Geometry: see drawing. Coordinates: mm, zero at the bounding-box minimum. A direction names the side the tool comes from. Coordinates: 2 decimals unless noted, no trailing zeros. Write each loop counter-clockwise with the first axis right and the second up, starting at its lowest first coordinate (ties: lowest second). Pieces come first, ordered by that corner, then holes. Notation, with made-up numbers: M 66.5,9.25 L 105.5,9.25 A31 ccw 105.5,38.25 Z; hole C 70,87 d10. An arc over 180 degrees is marked long. One line per item, written item: value. Start each with the question number.
Item 1: Cut plane B-B, the plane y = 17. Output: boundary loops of the cut face in (x, z), then the cut area to 3 significant figures.
Item 2: Mould query, pull axis Z, two halves, no side actions, for the marked faces 5, 6 and 7. Classes: released by +Z, released by -Z, zero draft, split by the parting line, or undercut.
Item 3: Set-up query: the marked faces 1, 2, 3 and 4. Return all of +Z, -Z, +X, -X, +Y, -Y with unobstructed straight access to the full face (end or side cutting, diameter ignored); none if empty.
Item 4: Cut plane A-A, the plane x = 26.5. Output: boundary loops of the cut face in (y, z) (1 decimal), then the cut area to 3 significant figures.
Item 5: Ray query, L1, parallel to X at y = 31, z = 6.5; L2, parallel to Z at x = 40, y = 4.5; L3, parallel to Y at x = 32, z = 41 (1 decimal). Return the intervals inside material, ascending. Write a range as from..to.
Item 6: Cut plane C-C, the plane z = 7. Output: boundary loops of the cut face in (x, y) (1 decimal), then the cut area to 3 significant figures.
Item 7: Cut plane D-D, the plane x = 7. Output: boundary loops of the cut face in (y, z), then the cut area to 3 significant figures.
Item 8: Pin query (flat end, axial travel): P1, Ø11, axis at x = 19.5, z = 40, coming from the -Y side; P2, Ø11, axis at x = 16.5, z = 40.5, coming from the +Y side (1 decimal); P3, Ø2.5, axis at y = 20.5, z = 37.5, coming from the -X side. Return the tip coordinate at first contact, or that it passes through.
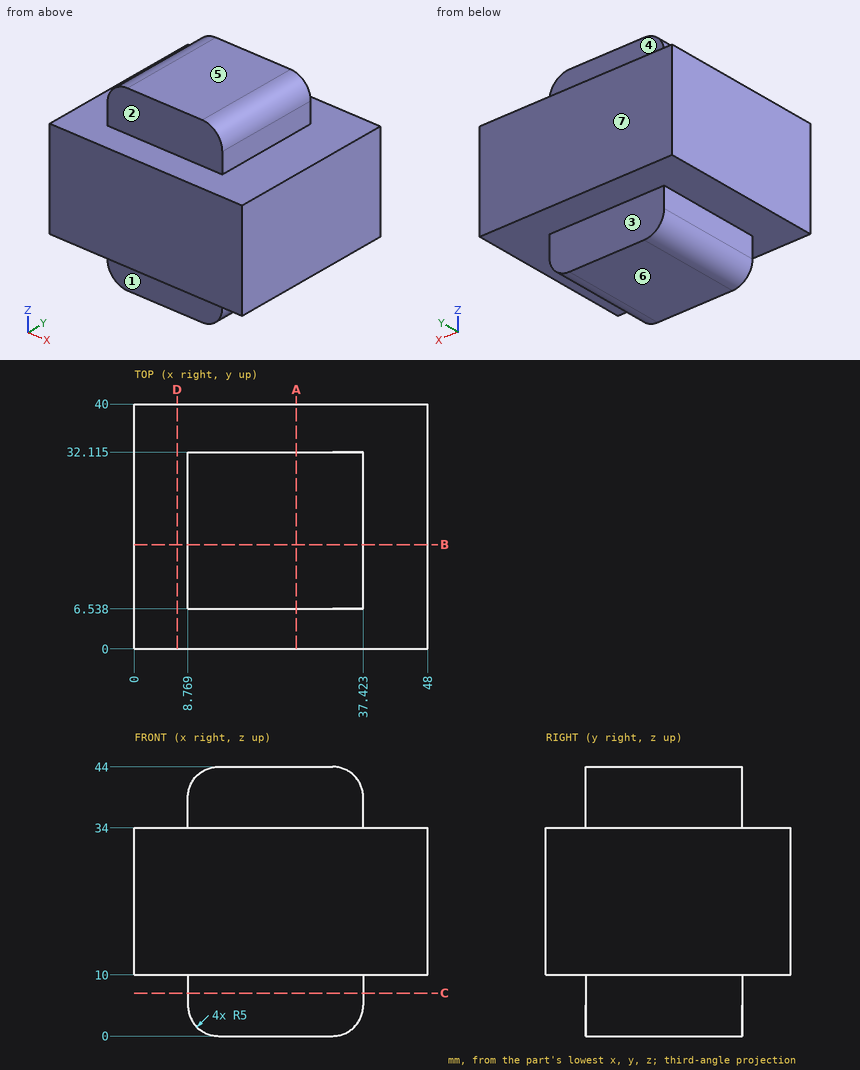
From the geometry:
1. outline: M 0,10 L 8.77,10 L 8.77,5 A5 ccw 13.77,0 L 32.42,0 A5 ccw 37.42,5 L 37.42,10 L 48,10 L 48,34 L 37.42,34 L 37.42,39 A5 ccw 32.42,44 L 13.77,44 A5 ccw 8.77,39 L 8.77,34 L 0,34 Z
1. area: 1,700 mm²
2. face 5: released by +Z
2. face 6: released by -Z
2. face 7: zero draft
3. face 1: -Z, +X, -X, -Y
3. face 2: +Z, +X, -X, -Y
3. face 3: -Z, +X, -X, +Y
3. face 4: +Z, +X, -X, +Y
4. outline: M 0,10 L 6.5,10 L 6.5,0 L 32.1,0 L 32.1,10 L 40,10 L 40,34 L 32.1,34 L 32.1,44 L 6.5,44 L 6.5,34 L 0,34 Z
4. area: 1,470 mm²
5. L1: x = 8.77..37.42
5. L2: z = 10..34
5. L3: y = 6.5..32.1
6. outline: M 8.8,6.5 L 37.4,6.5 L 37.4,32.1 L 8.8,32.1 Z
6. area: 733 mm²
7. outline: M 0,10 L 40,10 L 40,34 L 0,34 Z
7. area: 960 mm²
8. P1: stops at y = 6.54
8. P2: stops at y = 32.1
8. P3: stops at x = 8.77
